Geometry: final body of the model. Coordinates: model frame, mm. Face numbers are marked on the shaded views. A direction names the side the tool comes from. Round coordinates to 2 decimals unless told otherwise and drop trailing zeros. Write each loop counter-clockwise with the first axis right and the second up, starting at its lowest first coordinate (ties: lowest second). Pieces come first, ordered by that corner, then holes. Notation, with made-up numbers: M 6.5,-5 L 28.5,-5 A16 cw 28.5,7 Z; hole C 46,88.5 d4. An arc over 180 degrees is marked long. Answer as CSV lines item,"result". Start each with the question number.
Q1. First-contact query: pin 1 (2.5 mm diameter, centred on y = 9.5, z = 3, fed in from +X); pin 2 (11 mm diameter, centred on x = 2.5, y = 9, fed in from +Z); pin 3 (1.8 mm diameter, centred on x = 22, z = 1, fed in from -Y). Flat tips, straight axial feed; report the tip coordinate or a pass-through.
Q2. Section query A-A on z = 1. Output: boundary loops of the cut face in (x, y), and give its area (3 significant figures).
Q3. Ray query, probe 1 along Z at (x, y) = (27, 9.75); probe 2 along Z at (x, y) = (42, 20.25); probe 3 along X at (y, z) = (7.5, 4.75). Return the intervals inside material, ascending.
Q4. Mould query, pull axis X, two halves, no side actions, for the marked faces 3, 4 and 5. Classes: pulls with the +X half, pulls with the -X half, needs draft (parallel to the pull), parting line crosses it, or undercut.
Q5. Section query D-D on x = 38. Output: boundary loops of the cut face in (y, z), and give its area (3 significant figures).
Q6. Reachability of the marked faces 1 and 2 from +Z, -Z, +X, -X, +Y, -Y: full face, straight path, thin tool, end or side. Return the list, or none.
Q7. Section query B-B on x = 49.5. Output: boundary loops of the cut face in (y, z), and give its area (3 significant figures).
Q8. Section query C-C on y = 2. Output: boundary loops of the cut face in (x, z), and give its area (3 significant figures).
```python
from build123d import *

# Parameters (mm, degrees)
SKETCH1_W                  = 52
SKETCH1_H                  = 23
SKETCH1_R                  = 1.1
EXT_PCB_DEPTH              = 1.5
SKETCH2_W                  = 11.1
SKETCH2_H                  = 10
EXT_USB_SOCKET_DEPTH       = 5
SKETCH3_W                  = 52
SKETCH3_H                  = 16
EXT_COMPONENTS_DEPTH       = 1.6
SKETCH4_W                  = 8
SKETCH4_H                  = 7
EXT_RESET_BUTTON_DEPTH     = 2.2
SKETCH4_3_R                = 2
EXT_RESET_BUTTON_PEG_DEPTH = 7
SKETCH5_W                  = 4.4
SKETCH5_H                  = 9.4
EXT_USB_PLUG_DEPTH         = 2
SKETCH6_W                  = 1.5
SKETCH6_H                  = 10
EXT_USB_SLOT_DEPTH         = 3.1
EXT_START                  = -1.5
SKETCH7_R                  = 1.1
EXT_MOUNTS_DEPTH           = 8.5


with BuildPart() as part:
    # Sketch1 → ext PCB (new body)
    with BuildSketch(Plane.XY):
        with Locations((26, 11.5)):
            Rectangle(SKETCH1_W, SKETCH1_H)
        with Locations((2.5, 21)):
            Circle(SKETCH1_R, mode=Mode.SUBTRACT)
        with Locations((49.5, 21)):
            Circle(SKETCH1_R, mode=Mode.SUBTRACT)
        with Locations((2.5, 2)):
            Circle(SKETCH1_R, mode=Mode.SUBTRACT)
        with Locations((49.5, 2)):
            Circle(SKETCH1_R, mode=Mode.SUBTRACT)
    extrude(amount=-EXT_PCB_DEPTH)

    # Sketch2 → ext USB socket (add)
    with BuildSketch(Plane.XY):
        with Locations((4.45, 11.5)):
            Rectangle(SKETCH2_W, SKETCH2_H)
    extrude(amount=EXT_USB_SOCKET_DEPTH)

    # Sketch3 → ext Components (add)
    with BuildSketch(Plane.XY):
        with Locations((26, 11.5)):
            Rectangle(SKETCH3_W, SKETCH3_H)
    extrude(amount=EXT_COMPONENTS_DEPTH)

    # Sketch4 → ext Reset button (add)
    with BuildSketch(Plane.XY):
        with Locations((38, 14.5)):
            Rectangle(SKETCH4_W, SKETCH4_H)
    extrude(amount=EXT_RESET_BUTTON_DEPTH)

    # Sketch4<3> → ext Reset Button Peg (add)
    with BuildSketch(Plane.XY):
        with Locations((38, 14.5)):
            Circle(SKETCH4_3_R)
    extrude(amount=EXT_RESET_BUTTON_PEG_DEPTH)

    # Sketch5 → ext USB Plug (add)
    with BuildSketch(Plane.ZY.offset(1.1)):
        with Locations((2.5, 11.5)):
            Rectangle(SKETCH5_W, SKETCH5_H)
    extrude(amount=EXT_USB_PLUG_DEPTH)

    # Sketch6 → ext USB slot (add)
    with BuildSketch(Plane.ZY):
        Polygon((1.6, 6.5), (5, 6.5), (5, 16.5), (1.6, 16.5), (0, 16.5), (0, 6.5), align=None)
        with Locations((-0.75, 11.5)):
            Rectangle(SKETCH6_W, SKETCH6_H)
    extrude(amount=EXT_USB_SLOT_DEPTH)

    # Sketch7 → ext Mounts (add)
    with BuildSketch(Plane.XY.offset(EXT_START)):
        with Locations((49.5, 2)):
            Circle(SKETCH7_R)
        with Locations((2.5, 2)):
            Circle(SKETCH7_R)
        with Locations((2.5, 21)):
            Circle(SKETCH7_R)
        with Locations((49.5, 21)):
            Circle(SKETCH7_R)
    extrude(amount=EXT_MOUNTS_DEPTH)


solid = part.part
```
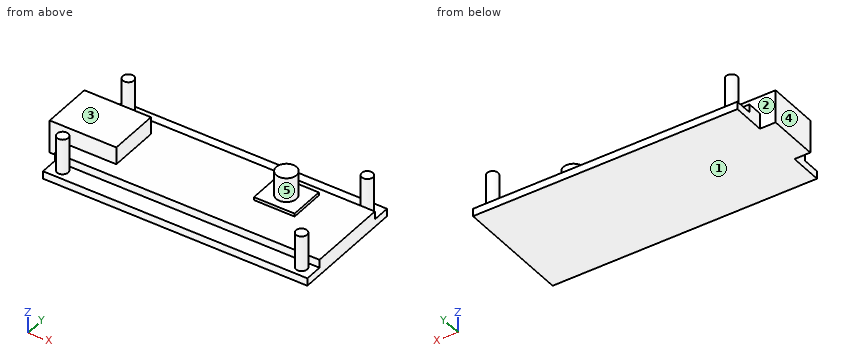
Entries:
1,pin 1,"stops at x = 10"
1,pin 2,"stops at z = 5"
1,pin 3,"stops at y = 3.5"
2,outline,"M -3.1,6.5 L 0,6.5 L 0,3.5 L 52,3.5 L 52,19.5 L 0,19.5 L 0,16.5 L -3.1,16.5 Z; C 2.5,2 d2.2; C 2.5,21 d2.2; C 49.5,2 d2.2; C 49.5,21 d2.2"
2,area,"878 mm^2"
3,probe 1,"z = -1.5 to 1.6"
3,probe 2,"z = -1.5 to 0"
3,probe 3,"x = -3.1 to 10"
4,face 3,"needs draft"
4,face 4,"pulls with the -X half"
4,face 5,"undercut"
5,outline,"M 0,-1.5 L 23,-1.5 L 23,0 L 19.5,0 L 19.5,1.6 L 18,1.6 L 18,2.2 L 16.5,2.2 L 16.5,7 L 12.5,7 L 12.5,2.2 L 11,2.2 L 11,1.6 L 3.5,1.6 L 3.5,0 L 0,0 Z"
5,area,"83.5 mm^2"
6,face 1,"-Z, +X, -X, +Y, -Y"
6,face 2,"+Z, -X"
7,outline,"M 0,-1.5 L 23,-1.5 L 23,0 L 22.1,0 L 22.1,7 L 19.9,7 L 19.9,0 L 19.5,0 L 19.5,1.6 L 3.5,1.6 L 3.5,0 L 3.1,0 L 3.1,7 L 0.9,7 L 0.9,0 L 0,0 Z"
7,area,"90.9 mm^2"
8,outline,"M 0,-1.5 L 52,-1.5 L 52,0 L 50.6,0 L 50.6,7 L 48.4,7 L 48.4,0 L 3.6,0 L 3.6,7 L 1.4,7 L 1.4,0 L 0,0 Z"
8,area,"109 mm^2"
